from build123d import *

# Parameters (mm, degrees)
F_120_X_74_PCB_OUTLINE_DEPTH               = 1.6
F_4_START                                  = -0.1
F_4_X_D3_2_PITCH_113_6_X_67_6_PROFILE_R    = 1.6
F_4_X_D3_2_PITCH_113_6_X_67_6_DEPTH        = 1.8
F_105_50_START                             = 1.55
F_105_50_X_67_20_LCD_MODULE_PROFILE_W      = 105.5
F_105_50_X_67_20_LCD_MODULE_PROFILE_H      = 67.2
F_105_50_X_67_20_LCD_MODULE_DEPTH          = 3.45
TOUCH_START                                = 4.98
TOUCH_PANEL_BLACK_BORDER_PROFILE_W         = 105.5
TOUCH_PANEL_BLACK_BORDER_PROFILE_H         = 67.2
TOUCH_PANEL_BLACK_BORDER_DEPTH             = 1.22
VISIBLE_START                              = 6.17
VISIBLE_480_X_272_DISPLAY_AREA_PROFILE_W   = 95.04
VISIBLE_480_X_272_DISPLAY_AREA_PROFILE_H   = 53.86
VISIBLE_480_X_272_DISPLAY_AREA_DEPTH       = 0.045
REAR_START                                 = -6
REAR_4_PIN_UART_CONNECTOR_HOUSING_PROFIL_W = 7.81
REAR_4_PIN_UART_CONNECTOR_HOUSING_PROFIL_H = 15.12
REAR_4_PIN_UART_CONNECTOR_HOUSING_DEPTH    = 6.05
UART_START                                 = -5.15
UART_CONNECTOR_SOCKET_PROFILE_W            = 5.9
UART_CONNECTOR_SOCKET_PROFILE_H            = 11.6
UART_CONNECTOR_SOCKET_DEPTH                = 3.9
REAR_START_2                               = -2
REAR_CARD_HOLDER_PROFILE_W                 = 14.85
REAR_CARD_HOLDER_PROFILE_H                 = 15
REAR_CARD_HOLDER_DEPTH                     = 2.05
CARD_START                                 = -1.77
CARD_OPENING_PROFILE_W                     = 12.4
CARD_OPENING_PROFILE_H                     = 8.7
CARD_OPENING_DEPTH                         = 0.9


with BuildPart() as part:
    # 120 x 74 PCB outline profile → 120 x 74 PCB outline (new body)
    with BuildSketch(Plane.XY):
        with BuildLine():
            Line((-56.8, -37), (56.8, -37))
            ThreePointArc((56.8, -37), (59.0627417, -36.0627417), (60, -33.8))
            Line((60, -33.8), (60, 33.8))
            ThreePointArc((60, 33.8), (59.0627417, 36.0627417), (56.8, 37))
            Line((56.8, 37), (-56.8, 37))
            ThreePointArc((-56.8, 37), (-59.0627417, 36.0627417), (-60, 33.8))
            Line((-60, 33.8), (-60, -33.8))
            ThreePointArc((-60, -33.8), (-59.0627417, -36.0627417), (-56.8, -37))
        make_face()
    extrude(amount=F_120_X_74_PCB_OUTLINE_DEPTH)

    # 4 x D3.2 - pitch 113.6 x 67.6 profile → 4 x D3.2 - pitch 113.6 x 67.6 (cut)
    with BuildSketch(Plane.XY.offset(F_4_START)):
        with Locations((-56.8, -33.8)):
            Circle(F_4_X_D3_2_PITCH_113_6_X_67_6_PROFILE_R)
        with Locations((-56.8, 33.8)):
            Circle(F_4_X_D3_2_PITCH_113_6_X_67_6_PROFILE_R)
        with Locations((56.8, -33.8)):
            Circle(F_4_X_D3_2_PITCH_113_6_X_67_6_PROFILE_R)
        with Locations((56.8, 33.8)):
            Circle(F_4_X_D3_2_PITCH_113_6_X_67_6_PROFILE_R)
    extrude(amount=F_4_X_D3_2_PITCH_113_6_X_67_6_DEPTH, mode=Mode.SUBTRACT)

    # 105.50 x 67.20 LCD module profile → 105.50 x 67.20 LCD module (add)
    with BuildSketch(Plane.XY.offset(F_105_50_START)):
        Rectangle(F_105_50_X_67_20_LCD_MODULE_PROFILE_W, F_105_50_X_67_20_LCD_MODULE_PROFILE_H)
    extrude(amount=F_105_50_X_67_20_LCD_MODULE_DEPTH)

    # Touch panel - black border profile → Touch panel - black border (add)
    with BuildSketch(Plane.XY.offset(TOUCH_START)):
        Rectangle(TOUCH_PANEL_BLACK_BORDER_PROFILE_W, TOUCH_PANEL_BLACK_BORDER_PROFILE_H)
    extrude(amount=TOUCH_PANEL_BLACK_BORDER_DEPTH)

    # Visible 480 x 272 display area profile → Visible 480 x 272 display area (add)
    with BuildSketch(Plane.XY.offset(VISIBLE_START)):
        with Locations((0, -1.23)):
            Rectangle(VISIBLE_480_X_272_DISPLAY_AREA_PROFILE_W, VISIBLE_480_X_272_DISPLAY_AREA_PROFILE_H)
    extrude(amount=VISIBLE_480_X_272_DISPLAY_AREA_DEPTH)

    # Rear 4-pin UART connector housing profile → Rear 4-pin UART connector housing (add)
    with BuildSketch(Plane.XY.offset(REAR_START)):
        with Locations((56.095, 0.04)):
            Rectangle(REAR_4_PIN_UART_CONNECTOR_HOUSING_PROFIL_W, REAR_4_PIN_UART_CONNECTOR_HOUSING_PROFIL_H)
    extrude(amount=REAR_4_PIN_UART_CONNECTOR_HOUSING_DEPTH)

    # UART connector socket profile → UART connector socket (cut)
    with BuildSketch(Plane.XY.offset(UART_START)):
        with Locations((57.25, 0.05)):
            Rectangle(UART_CONNECTOR_SOCKET_PROFILE_W, UART_CONNECTOR_SOCKET_PROFILE_H)
    extrude(amount=UART_CONNECTOR_SOCKET_DEPTH, mode=Mode.SUBTRACT)

    # Rear card holder profile → Rear card holder (add)
    with BuildSketch(Plane.XY.offset(REAR_START_2)):
        with Locations((-42.715, 29.5)):
            Rectangle(REAR_CARD_HOLDER_PROFILE_W, REAR_CARD_HOLDER_PROFILE_H)
    extrude(amount=REAR_CARD_HOLDER_DEPTH)

    # Card opening profile → Card opening (cut)
    with BuildSketch(Plane.XY.offset(CARD_START)):
        with Locations((-42.7, 32.85)):
            Rectangle(CARD_OPENING_PROFILE_W, CARD_OPENING_PROFILE_H)
    extrude(amount=CARD_OPENING_DEPTH, mode=Mode.SUBTRACT)


solid = part.part
Geometry: final body of the model. Coordinates: model frame, mm. A direction names the side the tool comes from. Give positions to 0.01 mm unless a question says otherwise; leave off trailing zeros. Loops run counter-clockwise (first coordinate to the right, second up) from the corner with the lowest first, then second, coordinate; pieces in that order, holes last. Notation, with made-up numbers: M 38,19.5 L 42,19.5 A17 cw 42,25.5 Z; hole C 78,70 d7. An arc over 180 degrees is marked long. Put each result on its own line as item: value. Start each with the question number.
1) Access query for faces 1 (the flat face through (-43, 33, -0.87)), 2 (the flat face through (54.3, 0, -3)), 3 (the flat face through (-1, -33.6, 4)). Directions: +Z, -Z, +X, -X, +Y, -Y. A direction counts if a zero-diameter tool reaches every point of the face in a straight line with its end or side. Return the directions, or none.
2) Cut plane C-C (z = -3.75). Output: boundary loops of the cut face in (x, y), then the cut area to 3 significant figures.
3) Cut plane B-B (x = 42). Output: boundary loops of the cut face in (y, z) (3 decimals), then the cut area to 3 significant figures.
4) Contact query for flat-ended pins moving along their axis: pin 1 (1.5 mm diameter, centred on x = -42, y = 29, fed in from -Z); pin 2 (1.7 mm diameter, centred on x = 57.5, y = -0.5, fed in from +Z); pin 3 (2 mm diameter, centred on x = -41.5, z = -1.5, fed in from -Y); pin 4 (5 mm diameter, centred on x = 3, z = 3.5, fed in from +Y). Output: stop coordinate, or through.
5) Cut plane D-D (y = 4). Output: boundary loops of the cut face in (x, z) (3 decimals), then the cut area to 3 significant figures.
6) Ray query, line 1 along X through (y, z) = (33.8, 1.15); line 2 along Y through (x, z) = (-56.8, 0.6); line 3 along Z through (x, y) = (-26, -20) (3 decimals). Return the intervals inside material, ascending.
7) Pull-direction query (X, two-part tool) for faces 4 (the flat face through (52.19, 0, -3)), 5 (the flat face through (56, -7.52, -3)), 6 (the cylindrical face through (55.2, 33.87, 0.79)); classes: pulls with the +X half, pulls with the -X half, needs draft (parallel to the pull), parting line crosses it, or undercut.
8) Cut plane A-A (y = 18). Output: boundary loops of the cut face in (x, z) (3 decimals), then the cut area to 3 significant figures.
Verdict:
1. face 1: +Y
1. face 2: +X
1. face 3: +Z, +X, -X, -Y
2. outline: M 52.19,-7.52 L 60,-7.52 L 60,-5.75 L 54.3,-5.75 L 54.3,5.85 L 60,5.85 L 60,7.6 L 52.19,7.6 Z
2. area: 52.0 mm2
3. outline: M -37,0 L 37,0 L 37,1.6 L 33.6,1.6 L 33.6,6.2 L 25.7,6.2 L 25.7,6.215 L -28.16,6.215 L -28.16,6.2 L -33.6,6.2 L -33.6,1.6 L -37,1.6 Z
3. area: 428 mm2
4. pin 1: z = -2
4. pin 2: z = 1.6
4. pin 3: y = 22
4. pin 4: y = 37
5. outline: M -60,0 L 52.19,0 L 52.19,-6 L 60,-6 L 60,-5.15 L 54.3,-5.15 L 54.3,-1.25 L 60,-1.25 L 60,1.6 L 52.75,1.6 L 52.75,6.2 L 47.52,6.2 L 47.52,6.215 L -47.52,6.215 L -47.52,6.2 L -52.75,6.2 L -52.75,1.6 L -60,1.6 Z
5. area: 703 mm2
6. line 1: -60 to -58.4, -55.2 to 55.2, 58.4 to 60
6. line 2: -37 to -35.4, -32.2 to 32.2, 35.4 to 37
6. line 3: 0 to 6.215
7. face 4: pulls with the -X half
7. face 5: needs draft
7. face 6: undercut
8. outline: M -60,0 L 60,0 L 60,1.6 L 52.75,1.6 L 52.75,6.2 L 47.52,6.2 L 47.52,6.215 L -47.52,6.215 L -47.52,6.2 L -52.75,6.2 L -52.75,1.6 L -60,1.6 Z
8. area: 679 mm2
